Here's how the part is built. I have some questions about the finished solid (model axes, mm). A direction names the side the tool comes from. Give positions to 0.01 mm unless a question says otherwise; leave off trailing zeros. Order: outer loops, then holes, each group sorted by start corner. A loop starts at its lowest first (then second) coordinate and runs counter-clockwise, first axis right, second up.
from build123d import *

# Parameters (mm, degrees)
MAIN_DEPTH      = 90
SKETCH2_R       = 1.25
SKETCH2_R_2     = 1.5
MAINHOLES_DEPTH = 6.5
SKETCH3_W       = 10
SKETCH3_H       = 55
PINHOLES_DEPTH  = 2


with BuildPart() as part:
    # Sketch1 → Main (new body)
    with BuildSketch(Plane.XY):
        Polygon((-5, 0), (5, 0), (5, -4.5), (1.45, -4.5), (1.45, -5.5), (-1.45, -5.5), (-1.45, -4.5), (-5, -4.5), align=None)
    extrude(amount=MAIN_DEPTH)

    # Sketch2 → MainHoles (cut, through all)
    with BuildSketch(Plane(origin=(0, 0, 0), x_dir=(1, 0, 0), z_dir=(0, 1, 0))):
        with Locations((0, -85)):
            Circle(SKETCH2_R)
        with Locations((0, -15)):
            Circle(SKETCH2_R)
        with Locations((0, -5)):
            Circle(SKETCH2_R_2)
    extrude(amount=-MAINHOLES_DEPTH, mode=Mode.SUBTRACT)

    # Sketch3 → PinHoles (cut)
    with BuildSketch(Plane(origin=(0, 0, 0), x_dir=(1, 0, 0), z_dir=(0, 1, 0))):
        with Locations((0, -50)):
            Rectangle(SKETCH3_W, SKETCH3_H)
    extrude(amount=-PINHOLES_DEPTH, mode=Mode.SUBTRACT)


solid = part.part
Q1. If we section it at A-A on y = -0.85: List the corners of the cut face in (x, z) for me, plus the area to 3 significant figures.
Filled sheet:
outline: (-5, 0) - (5, 0) - (5, 22.5) - (-5, 22.5) - close; (-5, 77.5) - (5, 77.5) - (5, 90) - (-5, 90) - close; hole circle Ø3 at (0, 5); hole circle Ø2.5 at (0, 15); hole circle Ø2.5 at (0, 85)
area: 333 mm2
Q2. If we section it at C-C on z = 85: List the corners of the cut face in (x, y) for me.
Filled sheet:
outline: (-5, -4.5) - (-1.45, -4.5) - (-1.45, -5.5) - (-1.25, -5.5) - (-1.25, 0) - (-5, 0) - close; (1.25, -5.5) - (1.45, -5.5) - (1.45, -4.5) - (5, -4.5) - (5, 0) - (1.25, 0) - close
Q3. I need wall thicknesses on L1, parallel to Z at x = 0, y = -3.7; L2, parallel to Z at x = 0, y = -1.2; L3, parallel to Z at x = 4, y = -1.1. Which ranges of each line are inside material? Lowest first, please.
Filled sheet:
L1: z = 0 to 3.5, 6.5 to 13.75, 16.25 to 83.75, 86.25 to 90
L2: z = 0 to 3.5, 6.5 to 13.75, 16.25 to 22.5, 77.5 to 83.75, 86.25 to 90
L3: z = 0 to 22.5, 77.5 to 90
Q4. I'm going to push flat-ended pins straight in: P1, Ø0.8, axis at y = -5, z = 1.5, coming from the +X side; P2, Ø0.8, axis at y = -5, z = 1.5, coming from the -X side; P3, Ø1.1, axis at x = 3, z = 47.5, coming from the -Y side. Where does each tip first touch, or does it pass through?
Filled sheet:
P1: stops at x = 1.45
P2: stops at x = -1.45
P3: stops at y = -4.5
Q5. For faces 4 (the face through (1, 0, 84)), 5 (the face through (0, -1, 22.5)), 6 (the face through (0, -2, 90)), 7 (the face through (-3, -4.5, 44)), 8 (the face through (3, -4.5, 44)), which set-ups out of +Z, -Z, +X, -X, +Y, -Y let a thin tool reach every point of the face, with its end or its side?
Filled sheet:
face 4: +Z, -Z, +X, -X, +Y
face 5: +X, -X, +Y
face 6: +Z, +X, -X, +Y, -Y
face 7: +Z, -Z, -X, -Y
face 8: +Z, -Z, +X, -Y
Q6. Thinking about a two-plate mould opening in X: for faces 1 (the face through (1.43, -2.71, 4.55)), 2 (the face through (-5, -3, 44)), 3 (the face through (0, -5.5, 47)), which applies, released by +X, released by -X, zero draft, split by the parting line, or undercut?
Filled sheet:
face 1: undercut
face 2: released by -X
face 3: zero draft
Q7. If we section it at B-B on x = 0: List the corners of the cut face in (y, z) for me, plus the area to 3 significant figures.
Filled sheet:
outline: (-5.5, 0) - (0, 0) - (0, 3.5) - (-5.5, 3.5) - close; (-5.5, 6.5) - (0, 6.5) - (0, 13.75) - (-5.5, 13.75) - close; (-5.5, 16.25) - (0, 16.25) - (0, 22.5) - (-2, 22.5) - (-2, 77.5) - (0, 77.5) - (0, 83.75) - (-5.5, 83.75) - close; (-5.5, 86.25) - (0, 86.25) - (0, 90) - (-5.5, 90) - close
area: 341 mm2
Q8. If we section it at D-D on z = 18: List the corners of the cut face in (x, y) for me, plus the area to 3 significant figures.
Filled sheet:
outline: (-5, -4.5) - (-1.45, -4.5) - (-1.45, -5.5) - (1.45, -5.5) - (1.45, -4.5) - (5, -4.5) - (5, 0) - (-5, 0) - close
area: 47.9 mm2
